Design review of the part built by this model. Coordinates are the model's own, in mm. Face numbers are marked on the shaded views. A direction names the side the tool comes from. Give positions to 0.01 mm unless a question says otherwise; leave off trailing zeros. Order: outer loops, then holes, each group sorted by start corner. A loop starts at its lowest first (then second) coordinate and runs counter-clockwise, first axis right, second up. Notation, with made-up numbers: (-35.5, -13.5) -> (-16.5, -13.5) arc R20 ccw to (-16.5, -1.5) -> close; hole circle Ø10 at (83, 59.5). An arc over 180 degrees is marked (long way). Return JSON: item names as keys, results as strings.
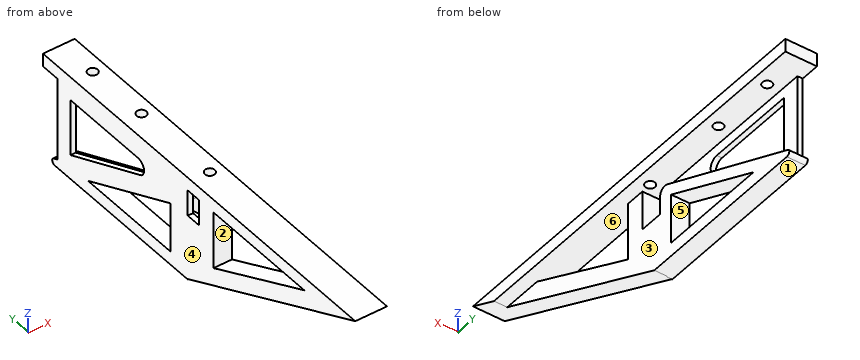
Autodesk Inventor part; units mm, degrees
ref_plane "Work Plane2" through (0, -97.663, -42.3664) normal (-1, 0, 0) x (0, 0, 1)
ref_plane "YZ Plane" through (0, 0, 0) normal (1, 0, 0) x (0, 1, 0)
ref_plane "XZ Plane" through (0, 0, 0) normal (0, 1, 0) x (-1, 0, 0)
ref_plane "Work Plane1" through (12.7, -42.953, -13.3823) normal (1, 0, 0) x (0, 1, 0)
sketch "Sketch1" plane through (12.7, -42.953, -13.3823) normal (1, 0, 0) x (0, 1, 0)
  line L0 (-54.71, 8.3023) -> (-54.71, 13.3823)
  line L1 (-54.71, 8.3023) -> (-47.0356, 8.3023)
  line L2 (-47.0356, 8.3023) -> (42.953, -31.0677)
  line L3 (42.953, -31.0677) -> (42.953, -10.5432)
  line L4 (42.953, -10.5432) -> (42.953, -7.1422)
  line L5 (42.953, -7.1422) -> (42.953, 13.3823)
  line L6 (42.953, 13.3823) -> (-54.71, 13.3823)
  line L7 (-18.8756, 8.3023) -> (29.7141, 8.3023)
  arc A0 (33.6511, 4.3653) -> (29.7141, 8.3023) centre (29.7141, 4.3653) ccw
  line L8 (33.6511, 4.3653) -> (33.6511, -16.8927)
  arc A1 (28.1361, -20.4997) -> (33.6511, -16.8927) centre (29.7141, -16.8927) ccw
  line L9 (28.1361, -20.4997) -> (-20.4536, 0.7583)
  arc A2 (-18.8756, 8.3023) -> (-20.4536, 0.7583) centre (-18.8756, 4.3653) ccw
  line L10 (-58.647, 13.3823) -> (-58.647, 8.3023)
  line L11 (-58.647, 13.3823) -> (-54.71, 13.3823)
  line L12 (-54.71, 8.3023) -> (-58.647, 8.3023)
  line L13 (42.953, 13.3823) -> (42.953, 19.7323)
  line L14 (42.953, 19.7323) -> (-160.247, 19.7323)
  line L15 (-160.247, 19.7323) -> (-50.8728, -31.0677)
  line L16 (-50.8728, -31.0677) -> (42.953, -31.0677)
  line L17 (42.953, -31.0677) -> (-47.0356, 8.3023)
  line L18 (-47.0356, 8.3023) -> (-47.0356, 0.7583)
  line L19 (-47.0356, 0.7583) -> (-58.647, 0.7583)
  line L20 (-58.647, 0.7583) -> (-58.647, 13.3823)
  line L21 (-58.647, 13.3823) -> (42.953, 13.3823)
  dimension "d0" = 6.35
  dimension "d1" = 203.2
ref_plane "Work Plane2" through (0, -97.663, -42.3664) normal (-1, 0, 0) x (0, 0, 1)
extrude "Extrusion1" add sketch "Sketch1" against normal up to surface (12.7 mm away) contours L11 L10 L20 L19 L18 L2 L16 L15 L14 L13 L6
sketch "Sketch2" plane through (12.7, -203.2, 6.35) normal (0, 0, 1) x (1, 0, 0)
  circle A0 centre (-6.35, 182.88) radius 2.3495
  circle A1 centre (-6.35, 151.13) radius 2.3495
  circle A2 centre (-6.35, 106.68) radius 2.3495
  point P0 (-12.7, 203.2)
extrude "Extrusion2" cut sketch "Sketch2" against normal blind 17.4625
sketch "Sketch3" plane through (0, -203.2, 6.35) normal (-1, 0, 0) x (0, 0, 1)
  line L0 (0, 203.2) -> (0, 0)
  line L1 (-6.35, 203.2) -> (0, 203.2)
  line L2 (-6.35, 101.6) -> (-6.35, 203.2)
  line L3 (-18.9739, 101.6) -> (-6.35, 101.6)
  line L4 (-18.9739, 113.2114) -> (-18.9739, 101.6)
  line L5 (-11.43, 113.2114) -> (-18.9739, 113.2114)
  line L6 (-50.8, 203.2) -> (-11.43, 113.2114)
  line L7 (-50.8, 109.3742) -> (-50.8, 203.2)
  line L8 (0, 0) -> (-50.8, 109.3742)
  line L9 (-35.8, 198.4375) -> (-35.8, 203.2)
  line L10 (-15.367, 193.8982) -> (-36.625, 193.8982)
  line L11 (0, 109.0295) -> (0, 104.3305)
  line L12 (-50.8, 193.8982) -> (0, 193.8982)
  line L13 (0, 193.8982) -> (0, 109.0295)
  line L14 (0, 109.0295) -> (-50.8, 109.0295)
  line L15 (-50.8, 109.0295) -> (-50.8, 193.8982)
extrude "Extrusion3" add sketch "Sketch3" along normal blind 2.54 contours L0 L12 L2 L1 | L0 L14 L2 L12 | L0 L8 L14 L4 L3 L2 | L2 L14 L4 L5 L6 L12 L10 | L14 L8 L7 L12 L6 L5 L4 | L14 L15 L8 | L12 L7 L6
sketch "Sketch4" plane through (0, -203.2, 6.35) normal (1, 0, 0) x (0, 0, -1)
  line L0 (11.43, 141.3714) -> (11.43, 189.9612)
  line L1 (11.43, 105.537) -> (6.35, 105.537)
  line L2 (11.43, 105.537) -> (11.43, 113.2114)
  line L3 (11.43, 113.2114) -> (50.8, 203.2)
  line L4 (50.8, 203.2) -> (30.2755, 203.2)
  line L5 (30.2755, 203.2) -> (26.8745, 203.2)
  line L6 (26.8745, 203.2) -> (6.35, 203.2)
  line L7 (6.35, 203.2) -> (6.35, 105.537)
  line L8 (11.43, 141.3714) -> (11.43, 189.9612)
  arc A0 (15.367, 193.8982) -> (11.43, 189.9612) centre (15.367, 189.9612) ccw
  line L9 (15.367, 193.8982) -> (36.625, 193.8982)
  arc A1 (40.2319, 188.3831) -> (36.625, 193.8982) centre (36.625, 189.9612) ccw
  line L10 (40.2319, 188.3831) -> (18.9739, 139.7934)
  arc A2 (11.43, 141.3714) -> (18.9739, 139.7934) centre (15.367, 141.3714) ccw
  line L11 (11.43, 185.3087) -> (38.8868, 185.3087)
extrude "Extrusion4" cut sketch "Sketch4" against normal blind 2.54 contours L0 L11 L10 A2
fillet "Fillet1" radius 3.175 1 edges at (6.35, -89.9886, -5.08)
fillet "Fillet2" radius 1.5875 1 edges at (5.08, 0, -44.45)
sketch "Sketch5" plane through (12.7, -42.953, -13.3823) normal (1, 0, 0) x (0, 0, -1)
  arc A0 (31.0677, 35.3637) -> (28.0258, 36) centre (29.4802, 35.3637) ccw
  line L0 (28.0258, 36) -> (-6.3564, -42.588)
  arc A1 (-6.3564, -42.588) -> (-3.4476, -47.0356) centre (-3.4476, -43.8606) ccw
  line L1 (-3.4476, -47.0356) -> (-0.7583, -47.0356)
  line L2 (-0.7583, -47.0356) -> (-0.7583, -58.647)
  line L3 (-0.7583, -58.647) -> (-13.3823, -58.647)
  line L4 (-13.3823, -58.647) -> (-13.3823, 42.953)
  line L5 (-13.3823, 42.953) -> (-19.7323, 42.953)
  line L6 (-19.7323, 42.953) -> (-19.7323, -160.247)
  line L7 (-19.7323, -160.247) -> (31.0677, -50.8728)
  line L8 (31.0677, -50.8728) -> (31.0677, 35.3637)
  line L9 (-13.3823, -127.1164) -> (-13.3823, -67.9876)
  line L10 (-13.3823, -127.1164) -> (14.3959, -67.9876)
  line L11 (14.3959, -67.9876) -> (-13.3823, -67.9876)
  line L12 (2.8311, -39.9014) -> (24.5341, -39.9014)
  line L13 (24.5341, -39.9014) -> (24.5341, 13.7178)
  line L14 (24.5341, 13.7178) -> (0.5068, -39.9014)
  line L15 (0.5068, -39.9014) -> (2.8311, -39.9014)
extrude "Extrusion5" cut sketch "Sketch5" against normal blind 17.78 contours L9 L11 L10 | L15 L14 L13 L12
chamfer "Chamfer1" distance 12.7 angle 45 1 edges at (12.7, -95.7943, -12.6239)
ref_plane "Work Plane3" through (6.35, 0, 0) normal (0, -1, 0) x (1, 0, 0)
sketch "Sketch6" plane through (12.7, -110.9406, -27.7782) normal (0, -1, 0) x (1, 0, 0)
  line L0 (-15.24, 34.1282) -> (-15.24, 27.7782)
  line L1 (-15.24, 34.1282) -> (-15.24, 27.7782)
  line L2 (0, 27.7782) -> (0, 0)
  line L3 (0, -16.6718) -> (-12.7, -16.6718)
  line L4 (0, 27.7782) -> (-6.35, 27.7782)
  line L5 (-6.35, 27.7782) -> (-6.35, -16.6718)
  line L6 (-6.35, -16.6718) -> (0, -16.6718)
  line L7 (0, -16.6718) -> (0, 27.7782)
  point P0 (-12.7, 27.7782)
  dimension "d17" = 6.35
  dimension "d18" = 6.35
extrude "Extrusion6" cut sketch "Sketch6" along normal mid plane 211.455
properties part number "PlateSpacer"
Item 1: Add section B-B (y = -113). Give the boundary of the cut face in (x, z), plus the area to 3 significant figures.
Result set:
{"outline": "(-2.54, -35.54) -> (6.35, -35.54) -> (6.35, -26.81) -> (-2.54, -26.81) -> close; (-2.54, 0) -> (12.7, 0) -> (12.7, 6.35) -> (-2.54, 6.35) -> close", "area": "174 mm^2"}
Item 2: Machinability: for the marked faces 3, 4, 5 and 6, which of the approach directions +Z, -Z, +X, -X, +Y, -Y give a long, thin tool a straight path to every point of the face, cutting with its end or side? Answer none if there is none.
Result set:
{"face 3": "-Z, +X, +Y, -Y", "face 4": "+Z, -Z, -X, +Y, -Y", "face 5": "+X, -X", "face 6": "+X"}
Item 3: Wall thickness on L1, parallel to Y at x = 6.35, z = 4.5; L2, parallel to Z at x = 4.5, y = -46.5; L3, parallel to Y at x = 4.25, z = -25: over which ranges is each line inside the solid? List them lowest first. Write a range as [from, to].
Result set:
{"L1": "y = [-199.22, -98.87], [-94.17, -54.42], [-49.72, -22.67], [-17.97, 0]", "L2": "z = [-44.45, -37.92], [-30.18, -24.11], [0, 6.35]", "L3": "y = [-135.7, -116.85], [-110.94, -82.85], [-58.06, -44.46]"}
Item 4: Add section D-D (y = -134). Give the boundary of the cut face in (x, z).
Result set:
{"outline": "(-2.54, -25.79) -> (6.35, -25.79) -> (6.35, -16.95) -> (-2.54, -16.95) -> close; (-2.54, 0) -> (12.7, 0) -> (12.7, 6.35) -> (-2.54, 6.35) -> close"}
Item 5: For pin 1 (0.8 mm diameter, centred on x = -1.5, z = -18, fed in from -Y); pin 2 (2.5 mm diameter, centred on x = 0, z = -6, fed in from +Y); pin 3 (2 mm diameter, centred on y = -35, z = -36.5, fed in from -X); pin 4 (1.5 mm diameter, centred on x = -0.5, y = -122, fed in from -Z), all flat-tipped, find the tip position at first contact; note any pin that passes through.
Result set:
{"pin 1": "stops at y = -151.63", "pin 2": "stops at y = -9.3", "pin 3": "passes through", "pin 4": "stops at z = -31.71"}
Item 6: Add section C-C (x = 10.5). Give the boundary of the cut face in (y, z), plus the area to 3 significant figures.
Result set:
{"outline": "(-203.2, 6.35) -> (-189.53, 0) -> (0, 0) -> (0, 6.35) -> close", "area": "1,250 mm^2"}
Item 7: Mouldability with a two-part tool opening along Y and no side actions: class the marked faces 1 and 2 as released by +Y, released by -Y, zero draft, split by the parting line, or undercut.
Result set:
{"face 1": "zero draft", "face 2": "undercut"}
Item 8: Add section A-A (y = -42). Give the boundary of the cut face in (x, z) (3 decimals), plus the area to 3 significant figures.
Result set:
{"outline": "(-2.54, -44.45) -> (6.35, -44.45) -> (6.35, -37.916) -> (-2.54, -37.916) -> close; (-2.54, -32.196) -> (6.35, -32.196) -> (6.35, -26.075) -> (0, -26.075) -> (0, -21.989) -> (-2.54, -21.989) -> close; (-2.54, -5.08) -> (0, -5.08) -> (0, 0) -> (12.7, 0) -> (12.7, 6.35) -> (-2.54, 6.35) -> close", "area": "233 mm^2"}
